Check sheet for the modelled part. Datum: model origin and axes. Units: mm. A direction names the side the tool comes from. Give positions to 0.01 mm unless a question says otherwise; leave off trailing zeros. Order: outer loops, then holes, each group sorted by start corner. A loop starts at its lowest first (then second) coordinate and runs counter-clockwise, first axis right, second up. Notation, with made-up numbers: (77, 34) -> (124, 34) arc R34 ccw to (124, 68) -> close; hole circle Ø3 at (-7, 50.5). An arc over 180 degrees is marked (long way). Write each question's results on one line, items separated by ' | '.
from build123d import *

# Parameters (mm, degrees)
BOSS_EXTRUDE1_DEPTH      = 15
BOSS_EXTRUDE2_DEPTH      = 15
BOSS_EXTRUDE3_DEPTH      = 192.8
BOSS_EXTRUDE4_DEPTH      = 7.5
BOSS_EXTRUDE4_DEPTH_BACK = 7.5
SKETCH5_R                = 38.1
SKETCH5_R_2              = 19.05
CUT_EXTRUDE1_DEPTH       = 2627.039580814
CUT_EXTRUDE2_DEPTH       = 15
CUT_EXTRUDE12_DEPTH      = 60
CUT_EXTRUDE16_DEPTH      = 2627.039580814
CUT_EXTRUDE16_DEPTH_BACK = 2627.039580814
SKETCH16_R               = 19.05
CUT_EXTRUDE17_DEPTH      = 2627.039580814
CUT_EXTRUDE17_DEPTH_BACK = 2627.039580814
SKETCH18_W               = 39.925079479
SKETCH18_H               = 106.526969349
CUT_EXTRUDE18_DEPTH      = 96.4


with BuildPart() as part:
    # Sketch1 → Boss-Extrude1 (new body)
    with BuildSketch(Plane.XY):
        Polygon((-2600, 304.8), (-2498.4, 304.8), (0, 254), (0, 0), (-177.8, 0), (-2498.4, 203.2), (-2600, 203.2), align=None)
    extrude(amount=-BOSS_EXTRUDE1_DEPTH)



with BuildPart() as body_2:
    # Sketch2 → Boss-Extrude2 (new body)
    with BuildSketch(Plane.XY.offset(177.8)):
        Polygon((-2498.4, 203.2), (-177.8, 0), (0, 0), (0, 254), (-2498.4, 304.8), (-2600, 304.8), (-2600, 203.2), align=None)
    extrude(amount=BOSS_EXTRUDE2_DEPTH)


with BuildPart() as part_1:
    add(part.part)

    add(body_2.part)  # Boss-Extrude3 merges body 2
    # Sketch3 → Boss-Extrude3 (add)
    with BuildSketch(Plane.XY.offset(192.8)):
        Polygon((-2600, 289.8), (-2600, 304.8), (-2498.4, 304.8), (0, 254), (0, 238.996899585), (-15, 239.301894782), (-2498.55248184, 289.8), align=None)
    extrude(amount=-BOSS_EXTRUDE3_DEPTH)

    # Sketch6 → Boss-Extrude4 (add, two sides: drawn at the far end of the back side and taken through both)
    with BuildSketch(Plane.XY.offset(88.9).offset(-BOSS_EXTRUDE4_DEPTH_BACK)):
        Polygon((-2498.4, 203.2), (-177.8, 0), (0, 0), (0, 254), (-2498.4, 304.8), (-2600, 304.8), (-2600, 203.2), align=None)
    extrude(amount=BOSS_EXTRUDE4_DEPTH + BOSS_EXTRUDE4_DEPTH_BACK)

    # Sketch5 → Cut-Extrude1 (cut, through all)
    with BuildSketch(Plane.XY.offset(192.8)):
        with Locations((-63.5, 176.782795882)):
            Circle(SKETCH5_R)
        with Locations((-171.45, 44.45)):
            Circle(SKETCH5_R_2)
    extrude(amount=-CUT_EXTRUDE1_DEPTH, mode=Mode.SUBTRACT)

    # Sketch7 → Cut-Extrude2 (cut)
    with BuildSketch(Plane.XY.offset(96.4)):
        Polygon((-1265.58125, 95.25), (0, 95.25), (0, 0), (-177.8, 0), align=None)
    extrude(amount=-CUT_EXTRUDE2_DEPTH, mode=Mode.SUBTRACT)

    # Sketch13 → Cut-Extrude12 (cut)
    with BuildSketch(Plane(origin=(0, 0, 81.4), x_dir=(-1, 0, 0), z_dir=(0, 0, -1))):
        Polygon((2605.267563799, 259.022933261), (2605.624161029, 249.594727716), (2612.822921274, 133.887362854), (1105.756685281, 0), (1095.76383028, 0), (1095.76383028, 94.872046381), (1091.720431016, 201.776969349), (1249.091648094, 207.729124269), align=None)
    extrude(amount=-CUT_EXTRUDE12_DEPTH, mode=Mode.SUBTRACT)

    # Sketch16 → Cut-Extrude16 (cut, two sides: drawn at the far end of the back side and taken through both)
    with BuildSketch(Plane(origin=(0, 0, -15), x_dir=(-1, 0, 0), z_dir=(0, 0, -1)).offset(-CUT_EXTRUDE16_DEPTH_BACK)):
        with Locations((1135.45885, 127.8123918)):
            Circle(SKETCH16_R)
    extrude(amount=CUT_EXTRUDE16_DEPTH + CUT_EXTRUDE16_DEPTH_BACK, mode=Mode.SUBTRACT)

    # Sketch17 → Cut-Extrude17 (cut, two sides: drawn at the far end of the back side and taken through both)
    with BuildSketch(Plane(origin=(0, 0, -15), x_dir=(-1, 0, 0), z_dir=(0, 0, -1)).offset(-CUT_EXTRUDE17_DEPTH_BACK)):
        with BuildLine():
            Line((1133.797122541, 146.789777338), (1761.395699383, 201.744543697))
            ThreePointArc((1761.395699383, 201.744543697), (1782.03481238, 184.428885618), (1764.719154301, 163.789772622))
            Line((1764.719154301, 163.789772622), (1137.120577459, 108.835006262))
            ThreePointArc((1137.120577459, 108.835006262), (1116.481464462, 126.150664341), (1133.797122541, 146.789777338))
        make_face()
    extrude(amount=CUT_EXTRUDE17_DEPTH + CUT_EXTRUDE17_DEPTH_BACK, mode=Mode.SUBTRACT)

    # Sketch18 → Cut-Extrude18 (cut)
    with BuildSketch(Plane(origin=(0, 0, 81.4), x_dir=(-1, 0, 0), z_dir=(0, 0, -1))):
        with Locations((1071.757891277, 148.513484675)):
            Rectangle(SKETCH18_W, SKETCH18_H)
        Polygon((1110.039582386, 201.776969349), (1091.720431016, 201.776969349), (1095.749535172, 95.25), (1091.720431016, 95.25), (1091.720431016, 86.714646079), (1110.039582386, 86.714646079), align=None)
    extrude(amount=-CUT_EXTRUDE18_DEPTH, mode=Mode.SUBTRACT)


with BuildPart() as body_2_2:
    # of the pieces the cut leaves, the one that is kept (cut_extrude18_keep)
    add(part_1.part.solids().sort_by_distance((-2600, 304.8, -15))[0])


solid = body_2_2.part
1. Section check A-A on x = -1523. Record the cut outline in (y, z).
Verdict:
outline: (117.79, -15) -> (142.62, -15) -> (142.62, 0) -> (117.79, 0) -> close; (117.79, 177.8) -> (142.62, 177.8) -> (142.62, 192.8) -> (117.79, 192.8) -> close; (180.87, -15) -> (284.97, -15) -> (284.97, 192.8) -> (180.87, 192.8) -> (180.87, 177.8) -> (269.96, 177.8) -> (269.96, 96.4) -> (218.09, 96.4) -> (218.09, 81.4) -> (269.96, 81.4) -> (269.96, 0) -> (180.87, 0) -> close
2. Section check D-D on x = -678. Record the cut outline in (y, z).
Verdict:
outline: (43.8, -15) -> (267.79, -15) -> (267.79, 192.8) -> (43.8, 192.8) -> (43.8, 177.8) -> (252.78, 177.8) -> (252.78, 96.4) -> (95.25, 96.4) -> (95.25, 81.4) -> (252.78, 81.4) -> (252.78, 0) -> (43.8, 0) -> close
3. Section check B-B on x = -63.5. Record the cut outline in (y, z).
Verdict:
outline: (0, -15) -> (138.68, -15) -> (138.68, 0) -> (0, 0) -> close; (0, 177.8) -> (138.68, 177.8) -> (138.68, 192.8) -> (0, 192.8) -> close; (95.25, 81.4) -> (138.68, 81.4) -> (138.68, 96.4) -> (95.25, 96.4) -> close; (214.88, -15) -> (255.29, -15) -> (255.29, 192.8) -> (214.88, 192.8) -> (214.88, 177.8) -> (240.29, 177.8) -> (240.29, 96.4) -> (214.88, 96.4) -> (214.88, 81.4) -> (240.29, 81.4) -> (240.29, 0) -> (214.88, 0) -> close
4. Mould release check, pull along Z, two halves, no side actions. Record for faces 1 (the flat face through (-1029, 194, 96.4)), 2 (the flat face through (-1443.203, 173.882, 185.405)), 3 (the flat face through (-1029, 194, 81.4)), 4 (the flat face through (-993, 188, -15)): +Z half, -Z half, draft (parallel to the pull), parting line (faces both ways), or undercut.
Verdict:
face 1: undercut | face 2: draft | face 3: undercut | face 4: -Z half
5. Gauge pin test, flat ends, axial feed: pin 1 Ø23 at (x, y) = (-171.45, 44.45) entering from -Z; pin 2 Ø16.5 at (x, z) = (-1080, 92) entering from -Y; pin 3 Ø3 at (x, z) = (-2229, 82) entering from -Y; pin 4 Ø24.5 at (x, z) = (-2559.5, 46.5) entering from -Y. Record the tip position at first contact, or that the pin passes through.
Verdict:
pin 1: passes through | pin 2: stops at y = 201.78 | pin 3: stops at y = 244.73 | pin 4: stops at y = 289.8
6. Section check C-C on z = 142.5. Record the cut outline in (x, y), then the cut area to 3 significant figures.
Verdict:
outline: (-2600, 289.8) -> (-2498.55, 289.8) -> (0, 239) -> (0, 254) -> (-2498.4, 304.8) -> (-2600, 304.8) -> close | area: 39,000 mm^2
7. Access from +Z, -Z, +X, -X, +Y, -Y to the whole of each face (thin tool, end or side, straight path). Record for faces 5 (the flat face through (-1354.344, 103.022, 185.195)), 6 (the flat face through (-1455.313, 136.697, 185.405)), 7 (the flat face through (-993, 179, 0)).
Verdict:
face 5: +Z, -Z, -X, -Y | face 6: +Z, -Z | face 7: -X, -Y
8. Material ranges on probe 1 along Z at (x, y) = (-767, 232.5); probe 2 along Z at (x, y) = (-1421, 127); probe 3 along Y at (x, z) = (-63.5, 189), recorded low to high. Write a range as from..to.
Verdict:
probe 1: z = -15..0, 81.4..96.4, 177.8..192.8 | probe 2: z = -15..0, 177.8..192.8 | probe 3: y = 0..138.68, 214.88..255.29
